from build123d import *

# Parameters (mm, degrees)
ESQUISSE1_R          = 4.5
ESQUISSE1_R_2        = 3
BASE_EXTRUSION_DEPTH = 2
CHANFREIN1_SIZE      = 0.5
CHANFREIN2_SIZE      = 0.2


with BuildPart() as part:
    # Esquisse1 → Base-Extrusion (new, symmetric)
    with BuildSketch(Plane.XY):
        Circle(ESQUISSE1_R)
        Circle(ESQUISSE1_R_2, mode=Mode.SUBTRACT)
    extrude(amount=BASE_EXTRUSION_DEPTH, both=True)

    # Chanfrein1
    chanfrein1_edges = [part.edges().sort_by_distance(p)[0] for p in [
        (-4.5, 0, -2),
        (-4.5, 0, 2),
    ]]
    chamfer(chanfrein1_edges, length=CHANFREIN1_SIZE)

    # Chanfrein2
    chanfrein2_edges = [part.edges().sort_by_distance(p)[0] for p in [
        (-3, 0, -2),
        (-3, 0, 2),
    ]]
    chamfer(chanfrein2_edges, length=CHANFREIN2_SIZE)


solid = part.part
Part model, mm, in its own coordinate system. Coordinates: 2 decimals unless noted, no trailing zeros. Loops run counter-clockwise (first coordinate to the right, second up) from the corner with the lowest first, then second, coordinate; pieces in that order, holes last. Notation, with made-up numbers: (-33.5, -2.75) -> (6.5, -2.75) arc R8 ccw to (6.5, 10.25) -> close; hole circle Ø8 at (67.25, 76.25). An arc over 180 degrees is marked (long way). Use a Markdown table: item, result. Add a question column.
Item 1: Probe probe 1 along Y at (x, z) = (0, 0.25); probe 2 along X at (y, z) = (-2.75, 0); probe 3 along X at (y, z) = (2.5, 0.15). List the from-to ranges inside material, lowest first.
Item 2: Band-saw the part on A-A on y = 0. Write the cut outline in (x, z), plus the area to 3 significant figures.
Item 3: Flat gauge pins, fed straight in: P1, Ø1, axis at y = 1.5, z = 1.5, coming from the +X side; P2, Ø2, axis at x = -3, y = 3.5, coming from the -Z side; P3, Ø1, axis at x = -3, z = 1, coming from the +Y side. Where does each tip first touch, or does it go through?
Item 4: Band-saw the part on C-C on z = 0.05. Write the cut outline in (x, y).
Item 5: Pull direction Y, two halves, no side cores. Call faces 1 (the cylindrical face through (-3, 0, 0)), 2 (the flat face through (-2, 3, -2)), 3 (the cylindrical face through (-0.59, 4.46, 0.02)): +Y half, -Y half, draft (parallel to the pull), parting line (faces both ways), or undercut.
Geometry says:
| question | item | result |
|---|---|---|
| 1 | probe 1 | -4.5 to -3, 3 to 4.5 |
| 1 | probe 2 | -3.56 to -1.2, 1.2 to 3.56 |
| 1 | probe 3 | -3.74 to -1.66, 1.66 to 3.74 |
| 2 | outline | (-4.5, -1.5) -> (-4, -2) -> (-3.2, -2) -> (-3, -1.8) -> (-3, 1.8) -> (-3.2, 2) -> (-4, 2) -> (-4.5, 1.5) -> close; (3, -1.8) -> (3.2, -2) -> (4, -2) -> (4.5, -1.5) -> (4.5, 1.5) -> (4, 2) -> (3.2, 2) -> (3, 1.8) -> close |
| 2 | area | 11.4 mm² |
| 3 | P1 | x = 4.39 |
| 3 | P2 | z = -2 |
| 3 | P3 | y = 3.74 |
| 4 | outline | circle Ø9 at (0, 0); hole circle Ø6 at (0, 0) |
| 5 | face 1 | undercut |
| 5 | face 2 | draft |
| 5 | face 3 | parting line |
